```python
from build123d import *

# Parameters (mm, degrees)
SKETCH1_W           = 25
SKETCH1_H           = 140
BOSS_EXTRUDE1_DEPTH = 8
SKETCH2_R           = 2.5
CUT_EXTRUDE1_DEPTH  = 143.439460825
SKETCH3_R           = 2.5
CUT_EXTRUDE2_DEPTH  = 143.439460825


with BuildPart() as part:
    # Sketch1 → Boss-Extrude1 (new body)
    with BuildSketch(Plane(origin=(0, 0, 0), x_dir=(1, 0, 0), z_dir=(0, 1, 0))):
        with Locations((12.5, 70)):
            Rectangle(SKETCH1_W, SKETCH1_H)
    extrude(amount=BOSS_EXTRUDE1_DEPTH)

    # Sketch2 → Cut-Extrude1 (cut, through all)
    with BuildSketch(Plane(origin=(0, 8, 0), x_dir=(1, 0, 0), z_dir=(0, 1, 0))):
        with Locations(Location((15, 7, 0), (0, 0, 270))):
            Circle(SKETCH2_R)
        with Locations(Location((15, 20, 0), (0, 0, 270))):
            Circle(SKETCH2_R)
        with Locations(Location((15, 30, 0), (0, 0, 270))):
            Circle(SKETCH2_R)
        with Locations(Location((15, 40, 0), (0, 0, 270))):
            Circle(SKETCH2_R)
        with Locations(Location((15, 52.5, 0), (0, 0, 270))):
            Circle(SKETCH2_R)
    extrude(amount=-CUT_EXTRUDE1_DEPTH, mode=Mode.SUBTRACT)

    # Sketch3 → Cut-Extrude2 (cut, through all)
    with BuildSketch(Plane(origin=(0, 0, 0), x_dir=(-1, 0, 0), z_dir=(0, -1, 0))):
        with Locations(Location((-14.998416969, 67.499999916, 0), (0, 0, 90))):
            Circle(SKETCH3_R)
        with Locations(Location((-14.997923514, 79.999999907, 0), (0, 0, 90))):
            Circle(SKETCH3_R)
        with Locations(Location((-14.997645062, 89.999999903, 0), (0, 0, 90))):
            Circle(SKETCH3_R)
        with Locations(Location((-14.997495222, 99.999999902, 0), (0, 0, 90))):
            Circle(SKETCH3_R)
        with Locations(Location((-14.99739352, 109.999999901, 0), (0, 0, 90))):
            Circle(SKETCH3_R)
        with Locations(Location((-14.997327839, 119.999999901, 0), (0, 0, 90))):
            Circle(SKETCH3_R)
        with Locations(Location((-14.997270403, 132.999999901, 0), (0, 0, 90))):
            Circle(SKETCH3_R)
    extrude(amount=-CUT_EXTRUDE2_DEPTH, mode=Mode.SUBTRACT)


solid = part.part
```
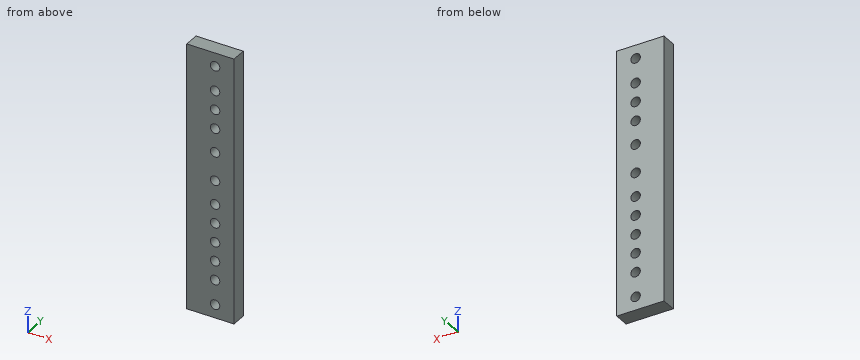
Design review of the part built by this model. Coordinates are the model's own, in mm. Round coordinates to 2 decimals unless told otherwise and drop trailing zeros. Order: outer loops, then holes, each group sorted by start corner. A loop starts at its lowest first (then second) coordinate and runs counter-clockwise, first axis right, second up. Notation, with made-up numbers: M -20.5,9.25 L 29.5,9.25 A9 cw 29.5,22.25 Z; hole C 28.25,-21.75 d1. An arc over 180 degrees is marked long. Put each result on its own line as item: value.
Q1. Consider section B-B (y = 4). State how many separate pieces and enclosed holes the cut face has, and give its area (3 significant figures).
Reported:
separate pieces: 1
enclosed holes: 12
area: 3,260 mm²
Q2. Consider section A-A (z = -7). State the section outline as (x, y) points, and give its area (3 significant figures).
Reported:
outline: M 0,0 L 12.5,0 L 12.5,8 L 0,8 Z; M 17.5,0 L 25,0 L 25,8 L 17.5,8 Z
area: 160 mm²
Q3. To check wall thickness, follow line 1 (X direction, y = 4.5, z = -80); line 2 (X direction, y = 4.75, z = -131). State the ranges of each line that lie inside material, in increasing order.
Reported:
line 1: 0 to 12.5, 17.5 to 25
line 2: 0 to 13.5, 16.5 to 25
Q4. Consider section C-C (z = -39.5). State the section outline as (x, y) points, and give its area (3 significant figures).
Reported:
outline: M 0,0 L 12.55,0 L 12.55,8 L 0,8 Z; M 17.45,0 L 25,0 L 25,8 L 17.45,8 Z
area: 161 mm²
Q5. Insertion check: pin 1 Ø4 at (x, z) = (15, -100) entering from -Y. The pin has a flat end and moves straight along its axis. Give the tip position at first contact, or say it passes through.
Reported:
pin 1: through
